Here's how the part is built. I have some questions about the finished solid (model axes, mm). A direction names the side the tool comes from. Give positions to 0.01 mm unless a question says otherwise; leave off trailing zeros. Loops run counter-clockwise (first coordinate to the right, second up) from the corner with the lowest first, then second, coordinate; pieces in that order, holes last. Notation, with made-up numbers: (48, -14) - (104, -14) arc R21 cw to (104, 12) - close; hole circle Ø2 at (-10.5, 72.5). An arc over 180 degrees is marked (long way). Use a Markdown table: item, result.
from build123d import *

# Parameters (mm, degrees)
SKETCH1_W           = 220
SKETCH1_H           = 95
BOSS_EXTRUDE1_DEPTH = 50
FILLET1_R           = 30
FILLET2_R           = 20
SHELL1_T            = -1.5


with BuildPart() as part:
    # Sketch1 → Boss-Extrude1 (new body)
    with BuildSketch(Plane.XY):
        with Locations((110, -47.5)):
            Rectangle(SKETCH1_W, SKETCH1_H)
    extrude(amount=BOSS_EXTRUDE1_DEPTH)

    # Fillet1
    fillet1_edges = [part.edges().sort_by_distance(p)[0] for p in [
        (0, 0, 25),
        (220, 0, 25),
        (220, -95, 25),
        (0, -95, 25),
    ]]
    fillet(fillet1_edges, radius=FILLET1_R)

    # Fillet2
    fillet2_edges = [part.edges().sort_by_distance(p)[0] for p in [
        (220, -47.5, 50),
        (110, -95, 50),
        (0, -47.5, 50),
        (110, 0, 50),
        (8.786796564, -8.786796564, 50),
        (8.786796564, -86.213203436, 50),
        (211.213203436, -8.786796564, 50),
        (211.213203436, -86.213203436, 50),
    ]]
    fillet(fillet2_edges, radius=FILLET2_R)

    # Shell1
    shell1_openings = [part.faces().sort_by_distance(p)[0] for p in [
        (110, -47.5, 0),
    ]]
    offset(amount=SHELL1_T, openings=shell1_openings, kind=Kind.INTERSECTION)


solid = part.part
(1) Will these pins go through, and if not, where does the flat tip stop? pin 1 (6 mm diameter, centred on y = -16, z = 9, fed in from -X); pin 2 (5 mm diameter, centred on y = -23, z = 35, fed in from +X); pin 3 (2 mm diameter, centred on y = -78.5, z = 33.5, fed in from +X).
A:
| item | result |
|---|---|
| pin 1 | x = 2.09 |
| pin 2 | x = 219.27 |
| pin 3 | x = 216.97 |
(2) On a 3-axis mill with a long thin cutter (end or side, diameter ignored), from which of +Z, -Z, +X, -X, +Y, -Y can I reach the whole of each face in a straight line? I mean faces 5 (the face through (109, -93.5, 15)), 6 (the face through (6.014, -47.745, 44.297)). Say none if no direction works.
A:
| item | result |
|---|---|
| face 5 | -Z |
| face 6 | +Z, -X, +Y, -Y |
(3) If I drill on line 1 (Y direction, x = 45, z = 15); line 2 (X direction, y = -39.5, z = 28.5); line 3 (Z direction, x = 33, y = -30), over which ranges is the centre line in solid material (lowest first)?
A:
| item | result |
|---|---|
| line 1 | -95 to -93.5, -1.5 to 0 |
| line 2 | 0 to 1.5, 218.5 to 220 |
| line 3 | 48.5 to 50 |
(4) We'd pull the mould along Y, two halves only. Please class faces 1 (the face through (210.4, -10.1, 15.2)), 2 (the face through (0, -48, 15)), 3 (the face through (109, 0, 15)), 4 (the face through (9.6, -84.9, 15.2)): pulls with the +Y half, pulls with the -Y half, needs draft (parallel to the pull), parting line crosses it, or undercut.
A:
| item | result |
|---|---|
| face 1 | undercut |
| face 2 | needs draft |
| face 3 | pulls with the +Y half |
| face 4 | undercut |
(5) Suppose I cut it at B-B on z = 12. Write out the boundary of the cut face in (x, y), plus the area to 3 significant figures.
A:
| item | result |
|---|---|
| outline | (0, -65) arc R30 ccw to (30, -95) - (190, -95) arc R30 ccw to (220, -65) - (220, -30) arc R30 ccw to (190, 0) - (30, 0) arc R30 ccw to (0, -30) - close; hole (1.5, -65) arc R28.5 ccw to (30, -93.5) - (190, -93.5) arc R28.5 ccw to (218.5, -65) - (218.5, -30) arc R28.5 ccw to (190, -1.5) - (30, -1.5) arc R28.5 ccw to (1.5, -30) - close |
| area | 861 mm2 |
(6) Suppose I cut it at C-C on x = 88.5. Write out the boundary of the cut face in (y, z), plus the area to 3 significant figures.
A:
| item | result |
|---|---|
| outline | (-95, 0) - (-93.5, 0) - (-93.5, 30) arc R18.5 cw to (-75, 48.5) - (-20, 48.5) arc R18.5 cw to (-1.5, 30) - (-1.5, 0) - (0, 0) - (0, 30) arc R20 ccw to (-20, 50) - (-75, 50) arc R20 ccw to (-95, 30) - close |
| area | 263 mm2 |
(7) Suppose I cut it at A-A on y = -42. Write out the boundary of the cut face in (x, z).
A:
| item | result |
|---|---|
| outline | (0, 0) - (1.5, 0) - (1.5, 30) arc R18.5 cw to (20, 48.5) - (200, 48.5) arc R18.5 cw to (218.5, 30) - (218.5, 0) - (220, 0) - (220, 30) arc R20 ccw to (200, 50) - (20, 50) arc R20 ccw to (0, 30) - close |
